Geometry: final body of the model. Coordinates: model frame, mm. A direction names the side the tool comes from. Give positions to 0.01 mm unless a question says otherwise; leave off trailing zeros. Write each loop counter-clockwise with the first axis right and the second up, starting at its lowest first coordinate (ties: lowest second). Pieces come first, ordered by that corner, then holes. Notation, with made-up numbers: (71.5, 58.5) -> (105.5, 58.5) arc R20 cw to (105.5, 95.5) -> close; hole circle Ø3 at (26.25, -3.75). An arc over 180 degrees is marked (long way). Answer as a JSON object with one key per item and string values.
from build123d import *

# Parameters (mm, degrees)
BOSS_EXTRUDE2_DEPTH  = 15
CUT_EXTRUDE1_DEPTH   = 13.5
SKETCH4_W            = 22
SKETCH4_H            = 1.5
CUT_EXTRUDE2_DEPTH   = 7.5
CUT_EXTRUDE3_DEPTH   = 1.5
CUT_EXTRUDE4_DEPTH   = 10
SKETCH21_W           = 1.5
SKETCH21_H           = 63.1126
BOSS_EXTRUDE6_DEPTH  = 13.5
CUT_EXTRUDE7_DEPTH   = 16
BOSS_EXTRUDE7_DEPTH  = 2
BOSS_EXTRUDE8_DEPTH  = 2
BOSS_EXTRUDE9_DEPTH  = 2
BOSS_EXTRUDE10_DEPTH = 9
SKETCH29_R           = 2.38125
CUT_EXTRUDE8_DEPTH   = 16
SKETCH31_R           = 2.38125
CUT_EXTRUDE9_DEPTH   = 6.35


with BuildPart() as part:
    # Sketch2 → Boss-Extrude2 (new body)
    with BuildSketch(Plane(origin=(0, 0, 0), x_dir=(1, 0, 0), z_dir=(0, 1, 0))):
        Polygon((40.1244, 0), (0, 0), (0, 66.1126), (64.116, 66.1126), (64.116, 23.9916), align=None)
        Polygon((41.6244, 1.5), (40.1244, 0), (64.116, 0), (52.1202, 11.9958), (51.059539828, 10.935139828), (60.494679656, 1.5), align=None)
    extrude(amount=BOSS_EXTRUDE2_DEPTH)

    # Sketch3 → Cut-Extrude1 (cut)
    with BuildSketch(Plane.XZ):
        Polygon((1.5, -64.6126), (62.616, -64.6126), (62.616, -24.612920344), (39.503079656, -1.5), (1.5, -1.5), align=None)
    extrude(amount=-CUT_EXTRUDE1_DEPTH, mode=Mode.SUBTRACT)

    # Sketch4 → Cut-Extrude2 (cut)
    with BuildSketch(Plane.XZ):
        with Locations((30.616, -65.3626)):
            Rectangle(SKETCH4_W, SKETCH4_H)
    extrude(amount=-CUT_EXTRUDE2_DEPTH, mode=Mode.SUBTRACT)

    # Sketch16 → Cut-Extrude3 (cut)
    with BuildSketch(Plane(origin=(0, 0, -66.1126), x_dir=(-1, 0, 0), z_dir=(0, 0, -1))):
        Polygon((-19.616, 0), (-9.616, 0), (-9.616, 9.5), (-54.116, 9.5), (-54.116, 0), (-41.616, 0), (-41.616, 7.5), (-19.616, 7.5), align=None)
    extrude(amount=-CUT_EXTRUDE3_DEPTH, mode=Mode.SUBTRACT)

    # Sketch18 → Cut-Extrude4 (cut)
    with BuildSketch(Plane(origin=(0, 15, 0), x_dir=(1, 0, 0), z_dir=(0, 1, 0))):
        with BuildLine():
            ThreePointArc((19.75, 66.1126), (16.5, 69.3626), (13.25, 66.1126))
            Line((13.25, 66.1126), (16.5, 66.1126))
            Line((16.5, 66.1126), (19.75, 66.1126))
        make_face()
        with BuildLine():
            Line((16.5, 66.1126), (13.25, 66.1126))
            ThreePointArc((13.25, 66.1126), (16.5, 62.8626), (19.75, 66.1126))
            Line((19.75, 66.1126), (16.5, 66.1126))
        make_face()
    extrude(amount=-CUT_EXTRUDE4_DEPTH, mode=Mode.SUBTRACT)

    # Sketch21 → Boss-Extrude6 (add)
    with BuildSketch(Plane.XZ):
        with Locations((3.75, -33.0563)):
            Rectangle(SKETCH21_W, SKETCH21_H)
    extrude(amount=-BOSS_EXTRUDE6_DEPTH)

    # Sketch24 → Cut-Extrude7 (cut, through all)
    with BuildSketch(Plane.XZ):
        Polygon((3, -1.5), (3, 0), (0, 0), (0, -66.1126), (3, -66.1126), align=None)
    extrude(amount=-CUT_EXTRUDE7_DEPTH, mode=Mode.SUBTRACT)

    # Sketch25 → Boss-Extrude7 (add)
    with BuildSketch(Plane.XZ):
        with BuildLine():
            Line((62.116, -70.1126), (62.116, -66.1126))
            Line((62.116, -66.1126), (58.116, -66.1126))
            Line((58.116, -66.1126), (54.116, -66.1126))
            Line((54.116, -66.1126), (54.116, -70.1126))
            ThreePointArc((54.116, -70.1126), (58.116, -74.1126), (62.116, -70.1126))
        make_face()
    extrude(amount=-BOSS_EXTRUDE7_DEPTH)

    # Sketch26 → Boss-Extrude8 (add)
    with BuildSketch(Plane.XZ):
        with BuildLine():
            Line((64.116, -51.1126), (64.116, -55.1126))
            Line((64.116, -55.1126), (68.116, -55.1126))
            ThreePointArc((68.116, -55.1126), (72.116, -51.1126), (68.116, -47.1126))
            Line((68.116, -47.1126), (64.116, -47.1126))
            Line((64.116, -47.1126), (64.116, -51.1126))
        make_face()
    extrude(amount=-BOSS_EXTRUDE8_DEPTH)

    # Sketch27 → Boss-Extrude9 (add)
    with BuildSketch(Plane.XZ):
        with BuildLine():
            ThreePointArc((63.774954249, -17.9937), (63.774954249, -12.336845751), (58.1181, -12.336845751))
            Line((58.1181, -12.336845751), (55.289672875, -15.165272875))
            Line((55.289672875, -15.165272875), (58.1181, -17.9937))
            Line((58.1181, -17.9937), (60.946527125, -20.822127125))
            Line((60.946527125, -20.822127125), (63.774954249, -17.9937))
        make_face()
    extrude(amount=-BOSS_EXTRUDE9_DEPTH)

    # Sketch28 → Boss-Extrude10 (add)
    with BuildSketch(Plane.XZ):
        with BuildLine():
            Line((-1, -55.1126), (3, -55.1126))
            Line((3, -55.1126), (3, -51.1126))
            Line((3, -51.1126), (3, -47.1126))
            Line((3, -47.1126), (-1, -47.1126))
            ThreePointArc((-1, -47.1126), (-5, -51.1126), (-1, -55.1126))
        make_face()
    extrude(amount=-BOSS_EXTRUDE10_DEPTH)

    # Sketch29 → Cut-Extrude8 (cut, through all)
    with BuildSketch(Plane.XZ):
        with Locations((60.946527125, -15.165272875)):
            Circle(SKETCH29_R)
        with Locations((68.116, -51.1126)):
            Circle(SKETCH29_R)
        with Locations((58.116, -70.1126)):
            Circle(SKETCH29_R)
    extrude(amount=-CUT_EXTRUDE8_DEPTH, mode=Mode.SUBTRACT)

    # Sketch31 → Cut-Extrude9 (cut)
    with BuildSketch(Plane.XZ):
        with Locations((-1, -51.1126)):
            Circle(SKETCH31_R)
    extrude(amount=-CUT_EXTRUDE9_DEPTH, mode=Mode.SUBTRACT)


solid = part.part
Q1. Cut plane C-C (y = 10.5). Return the cut outline in (x, z), and give its area (3 significant figures).
Values:
{"outline": "(3, -66.11) -> (13.25, -66.11) arc R3.25 cw to (13.62, -64.61) -> (4.5, -64.61) -> (4.5, -1.5) -> (39.5, -1.5) -> (62.62, -24.61) -> (62.62, -64.61) -> (19.38, -64.61) arc R3.25 cw to (19.75, -66.11) -> (64.12, -66.11) -> (64.12, -23.99) -> (52.12, -12) -> (64.12, 0) -> (3, 0) -> close; hole (41.62, -1.5) -> (51.06, -10.94) -> (60.49, -1.5) -> close", "area": "397 mm²"}
Q2. Cut plane B-B (x = 35.5). Return the cut outline in (y, z), and give its area (3 significant figures).
Values:
{"outline": "(0, -1.5) -> (13.5, -1.5) -> (13.5, -64.61) -> (9.5, -64.61) -> (9.5, -66.11) -> (15, -66.11) -> (15, 0) -> (0, 0) -> close", "area": "125 mm²"}
Q3. Cut plane D-D (x = 47). Return the cut outline in (y, z), and give its area (3 significant figures).
Values:
{"outline": "(0, -9) -> (13.5, -9) -> (13.5, -64.61) -> (9.5, -64.61) -> (9.5, -66.11) -> (15, -66.11) -> (15, -6.88) -> (0, -6.88) -> close; (0, -1.5) -> (15, -1.5) -> (15, 0) -> (0, 0) -> close", "area": "146 mm²"}
Q4. Set-up query: faces 5 (the flat face through (62.34, 0.99, -19.43)), 6 (the cylindrical face through (16.429, 14.122, -62.863)), 7 (the flat face through (66, 1, -55.113)), 8 (the flat face through (34, 15, -34)), 9 (the cylindrical face through (-1.31, 3.13, -48.75)). Return all of +Z, -Z, +X, -X, +Y, -Y with unobstructed straight access to the full face (end or side cutting, diameter ignored); none if empty.
Values:
{"face 5": "+X, +Y, -Y", "face 6": "-Z, +Y, -Y", "face 7": "-Z, +X, +Y, -Y", "face 8": "+Z, -Z, +X, -X, +Y", "face 9": "-Y"}
Q5. Cut plane A-A (z = -44). Return the cut outline in (x, y).
Values:
{"outline": "(3, 0) -> (4.5, 0) -> (4.5, 13.5) -> (62.62, 13.5) -> (62.62, 0) -> (64.12, 0) -> (64.12, 15) -> (3, 15) -> close"}
Q6. Material intervals for L1, parallel to X at y = 7, z = -61; L2, parallel to Y at x = 42.5, z = -22; L3, parallel to Z at x = 37.5, y = 11.5, sorted ascending. Write a range as from..to.
Values:
{"L1": "3..4.5, 62.62..64.12", "L2": "13.5..15", "L3": "-66.11..-64.61, -1.5..0"}
Q7. First-contact query: P1, Ø1.2, axis at y = 4, z = -65, coming from the +X side; P2, Ø5, axis at x = 59.5, y = 12, coming from the -Z side; P3, Ø1.7, axis at x = 32, z = -65.5, coming from the -Y side. Flat tips, straight axial feed; report the tip coordinate or a pass-through.
Values:
{"P1": "x = 64.12", "P2": "z = -66.11", "P3": "y = 9.5"}
Q8. Mould query, pull axis X, two halves, no side actions, for faces 1 (the flat face through (4.5, 7, -33)), 2 (the flat face through (1, 4, -55.113)), 3 (the cylindrical face through (-5, 4, -51)), 4 (the flat face through (56.724, 0.986, -13.731)). Classes: pulls with the +X half, pulls with the -X half, needs draft (parallel to the pull), parting line crosses it, or undercut.
Values:
{"face 1": "undercut", "face 2": "needs draft", "face 3": "pulls with the -X half", "face 4": "undercut"}
